```python
from build123d import *

# Parameters (mm, degrees)
SKETCH1_W           = 101.6
SKETCH1_H           = 25.4
BOSS_EXTRUDE1_DEPTH = 215.9
SKETCH2_R           = 5.08
BOSS_EXTRUDE2_DEPTH = 17.78
SKETCH3_W           = 27.94
SKETCH3_H           = 47.346080225
CUT_EXTRUDE1_DEPTH  = 27.686
SKETCH9_W           = 45.72
SKETCH9_H           = 71.12
BOSS_EXTRUDE5_DEPTH = 45.72
CUT_EXTRUDE4_DEPTH  = 45.72
BOSS_EXTRUDE6_DEPTH = 25.4


with BuildPart() as part:
    # Sketch1 → Boss-Extrude1 (new body)
    with BuildSketch(Plane(origin=(0, 0, 0), x_dir=(1, 0, 0), z_dir=(0, 1, 0))):
        with Locations((29.457987906, 2.028993953)):
            Rectangle(SKETCH1_W, SKETCH1_H)
    extrude(amount=BOSS_EXTRUDE1_DEPTH)

    # Sketch2 → Boss-Extrude2 (add)
    with BuildSketch(Plane(origin=(0, 215.9, 0), x_dir=(1, 0, 0), z_dir=(0, 1, 0))):
        with Locations(Location((-1.022012094, 2.028993953, 0), (0, 0, 90))):
            Circle(SKETCH2_R)
        with Locations(Location((59.937987906, 2.028993953, 0), (0, 0, 90))):
            Circle(SKETCH2_R)
    extrude(amount=BOSS_EXTRUDE2_DEPTH)

    # Sketch3 → Cut-Extrude1 (cut)
    with BuildSketch(Plane.XY.offset(10.671006047)):
        with Locations((-7.372012094, 23.673040113)):
            Rectangle(SKETCH3_W, SKETCH3_H)
        with Locations((66.287987906, 23.673040113)):
            Rectangle(SKETCH3_W, SKETCH3_H)
    extrude(amount=-CUT_EXTRUDE1_DEPTH, mode=Mode.SUBTRACT)

    # Sketch9 → Boss-Extrude5 (add)
    with BuildSketch(Plane.XY.offset(10.671006047)):
        with Locations((29.457987906, 35.56)):
            Rectangle(SKETCH9_W, SKETCH9_H)
    extrude(amount=BOSS_EXTRUDE5_DEPTH)

    # Sketch10 → Cut-Extrude4 (cut)
    with BuildSketch(Plane(origin=(52.317987906, 0, 0), x_dir=(0, 0, -1), z_dir=(1, 0, 0))):
        Polygon((-56.391006047, 71.12), (-10.671006047, 71.12), (-56.391006047, 0), align=None)
    extrude(amount=-CUT_EXTRUDE4_DEPTH, mode=Mode.SUBTRACT)

    # Sketch11 → Boss-Extrude6 (add)
    with BuildSketch(Plane(origin=(0, 0, -14.728993953), x_dir=(-1, 0, 0), z_dir=(0, 0, -1))):
        Polygon((-52.317987906, 47.346080225), (-52.317987906, 70.979374422), (-6.597987906, 70.979374422), (-6.597987906, 47.346080225), (-6.597987906, 0), (-52.317987906, 0), align=None)
    extrude(amount=BOSS_EXTRUDE6_DEPTH)


solid = part.part
```
Geometry check sheet. Reference: the model listing, model coordinates, mm. A direction names the side the tool comes from. Give positions to 0.01 mm unless a question says otherwise; leave off trailing zeros. Write each loop counter-clockwise with the first axis right and the second up, starting at its lowest first coordinate (ties: lowest second). Pieces come first, ordered by that corner, then holes. Notation, with made-up numbers: (-28, -39.5) - (-16, -39.5) arc R21 cw to (-16, -23.5) - close; hole circle Ø7 at (37.5, 38.25). An arc over 180 degrees is marked (long way). Use a Markdown table: item, result.
Q1. Section check D-D, the plane z = -31.5. Enter the section's corners in (x, y).
Computed:
| item | result |
|---|---|
| outline | (6.6, 0) - (52.32, 0) - (52.32, 70.98) - (6.6, 70.98) - close |
Q2. Section check C-C, the plane y = 171. Enter the section's corners in (x, z).
Computed:
| item | result |
|---|---|
| outline | (-21.34, -14.73) - (80.26, -14.73) - (80.26, 10.67) - (-21.34, 10.67) - close |
Q3. Go/stop test with flat-tipped pins: P1, Ø2, axis at x = 36, y = 184.5, coming from the -Z side; P2, Ø8, axis at x = 16, y = 85, coming from the +Z side; P3, Ø12, axis at x = 56, y = 31, coming from the +Z side. Record where each tip stops, or that it passes through.
Computed:
| item | result |
|---|---|
| P1 | stops at z = -14.73 |
| P2 | stops at z = 10.67 |
| P3 | stops at z = 39.51 |
Q4. Draft check along X on faces 1 (the face through (80.258, 130, -2)), 2 (the face through (-8, 47.346, -2)), 3 (the face through (3.937, 224.666, -0.928)). Enter one of: pulls with the +X half, pulls with the -X half, needs draft (parallel to the pull), parting line crosses it, or undercut.
Computed:
| item | result |
|---|---|
| face 1 | pulls with the +X half |
| face 2 | needs draft |
| face 3 | undercut |
Q5. Section check B-B, the plane x = 30.5. Enter the section's corners in (y, z).
Computed:
| item | result |
|---|---|
| outline | (0, -40.13) - (70.98, -40.13) - (70.98, -14.73) - (215.9, -14.73) - (215.9, 10.67) - (71.12, 10.67) - (0, 56.39) - close |
Q6. Set-up check for faces 4 (the face through (64.897, 224.666, -0.928)), 5 (the face through (30, 70.979, -27)), 6 (the face through (-1, 233.68, -2)), 7 (the face through (29.78, 36.06, 33.21)), 8 (the face through (66, 47.346, -2)): record each of +Z, -Z, +X, -X, +Y, -Y from which the full face is reachable in a straight line by a thin tool's end or side.
Computed:
| item | result |
|---|---|
| face 4 | +Y |
| face 5 | -Z, +X, -X, +Y |
| face 6 | +Z, -Z, +X, -X, +Y |
| face 7 | +Z, +X, -X, +Y |
| face 8 | +Z, -Z, +X, -Y |
Q7. Thickness scan on L1, parallel to X at y = 32, z = 26.5; L2, parallel to Z at x = -12, y = 134; L3, parallel to Y at x = 44, z = 3. Record the ranges inside material, lowest first. Write a range as [from, to].
Computed:
| item | result |
|---|---|
| L1 | x = [6.6, 52.32] |
| L2 | z = [-14.73, 10.67] |
| L3 | y = [0, 215.9] |
Q8. Section check A-A, the plane z = 6.5. Enter the section's corners in (x, y), then the cut area to 3 significant figures.
Computed:
| item | result |
|---|---|
| outline | (-21.34, 47.35) - (6.6, 47.35) - (6.6, 0) - (52.32, 0) - (52.32, 47.35) - (80.26, 47.35) - (80.26, 215.9) - (-21.34, 215.9) - close |
| area | 19,300 mm² |
